```python
from build123d import *

# Parameters (mm, degrees)
SKETCH1_R           = 63.5
SKETCH1_R_2         = 9
SKETCH1_R_3         = 2.5
BOSS_EXTRUDE1_DEPTH = 25.5
FILLET1_R           = 2


with BuildPart() as part:
    # Sketch1 → Boss-Extrude1 (new, symmetric)
    with BuildSketch(Plane.XY):
        Circle(SKETCH1_R)
        Circle(SKETCH1_R_2, mode=Mode.SUBTRACT)
        with Locations((0, 23.75)):
            Circle(SKETCH1_R_3, mode=Mode.SUBTRACT)
        with Locations((20.56810334, 11.875)):
            Circle(SKETCH1_R_3, mode=Mode.SUBTRACT)
        with Locations((20.56810334, -11.875)):
            Circle(SKETCH1_R_3, mode=Mode.SUBTRACT)
        with Locations((0, -23.75)):
            Circle(SKETCH1_R_3, mode=Mode.SUBTRACT)
        with Locations((-20.56810334, -11.875)):
            Circle(SKETCH1_R_3, mode=Mode.SUBTRACT)
        with Locations((-20.56810334, 11.875)):
            Circle(SKETCH1_R_3, mode=Mode.SUBTRACT)
    extrude(amount=BOSS_EXTRUDE1_DEPTH, both=True)

    # Fillet1
    fillet1_edges = [part.edges().sort_by_distance(p)[0] for p in [
        (-9, 0, -25.5),
        (-9, 0, 25.5),
    ]]
    fillet(fillet1_edges, radius=FILLET1_R)


solid = part.part
```
Verification items for the finished model (mm, model axes). Give positions to 0.01 mm unless a question says otherwise; leave off trailing zeros. Loops run counter-clockwise (first coordinate to the right, second up) from the corner with the lowest first, then second, coordinate; pieces in that order, holes last. Notation, with made-up numbers: M 12.5,50 L 33.5,50 A25 ccw 33.5,70 Z; hole C -36.75,24 d2. An arc over 180 degrees is marked long. One line per question, with ' | ' between items.
Item 1: Section check A-A, the plane y = 0. Record the cut outline in (x, z).
Completed:
outline: M -63.5,-25.5 L -11,-25.5 A2 ccw -9,-23.5 L -9,23.5 A2 ccw -11,25.5 L -63.5,25.5 Z; M 9,-23.5 A2 ccw 11,-25.5 L 63.5,-25.5 L 63.5,25.5 L 11,25.5 A2 ccw 9,23.5 Z
Item 2: Thickness scan on line 1 (Y direction, x = 0, z = 12); line 2 (X direction, y = 0.5, z = -1.5); line 3 (X direction, y = 5, z = 8). Record the ranges inside material, lowest first. Write a range as [from, to].
Completed:
line 1: y = [-63.5, -26.25], [-21.25, -9], [9, 21.25], [26.25, 63.5] | line 2: x = [-63.5, -8.99], [8.99, 63.5] | line 3: x = [-63.3, -7.48], [7.48, 63.3]
Item 3: Section check D-D, the plane y = -23.75. Record the cut outline in (x, z).
Completed:
outline: M -58.89,-25.5 L -2.5,-25.5 L -2.5,25.5 L -58.89,25.5 Z; M 2.5,-25.5 L 58.89,-25.5 L 58.89,25.5 L 2.5,25.5 Z
Item 4: Depth check by flat-ended pin: P1, Ø10, axis at x = -31.5, z = -15.5, coming from the +Y side; P2, Ø2, axis at y = 6, z = 18.5, coming from the +X side; P3, Ø8, axis at x = -29.5, z = 16, coming from the -Y side. Enter the tip coordinate at first touch or a pass-through.
Completed:
P1: stops at y = 57.71 | P2: stops at x = 63.3 | P3: stops at y = -58.15
Item 5: Section check C-C, the plane z = 21.5. Record the cut outline in (x, y) (3 decimals).
Completed:
outline: C 0,0 d127; hole C -20.568,-11.875 d5; hole C -20.568,11.875 d5; hole C 0,0 d18; hole C 0,-23.75 d5; hole C 0,23.75 d5; hole C 20.568,-11.875 d5; hole C 20.568,11.875 d5
Item 6: Section check B-B, the plane x = 0. Record the cut outline in (y, z), plus the area to 3 significant figures.
Completed:
outline: M -63.5,-25.5 L -26.25,-25.5 L -26.25,25.5 L -63.5,25.5 Z; M -21.25,-25.5 L -11,-25.5 A2 ccw -9,-23.5 L -9,23.5 A2 ccw -11,25.5 L -21.25,25.5 Z; M 9,-23.5 A2 ccw 11,-25.5 L 21.25,-25.5 L 21.25,25.5 L 11,25.5 A2 ccw 9,23.5 Z; M 26.25,-25.5 L 63.5,-25.5 L 63.5,25.5 L 26.25,25.5 Z | area: 5,050 mm^2
Item 7: Draft check along Y on faces 1 (the face through (-13.77, -61.99, 0.36)), 2 (the face through (13, 1, 25.5)), 3 (the face through (-22.55, -13.4, -0.36)), 4 (the face through (-1.172, 8.923, -0.329)). Enter one of: +Y half, -Y half, draft (parallel to the pull), parting line (faces both ways), or undercut.
Completed:
face 1: parting line | face 2: draft | face 3: undercut | face 4: undercut
